Could you check a few things on this model? Use its own coordinates, in mm. Give positions to 0.01 mm unless a question says otherwise; leave off trailing zeros. Write each loop counter-clockwise with the first axis right and the second up, starting at its lowest first coordinate (ties: lowest second). Pieces come first, ordered by that corner, then holes. Notation, with made-up numbers: (-27, 47) - (12, 47) arc R32 ccw to (12, 83) - close; hole circle Ø10 at (23.25, 56.25). An arc over 180 degrees is marked (long way). Answer as a JSON object with one key per item and string values. Group by question number.
```python
from build123d import *

# Parameters (mm, degrees)
ESQUISSE1_R        = 2
ESQUISSE1_R_2      = 1.5
BOSS_EXTRU_1_DEPTH = 2.5


with BuildPart() as part:
    # Esquisse1 → Boss.-Extru.1 (new body)
    with BuildSketch(Plane.XY):
        with BuildLine():
            Line((0, 0), (70, 0))
            Line((70, 0), (70, 10))
            Line((70, 10), (0, 10))
            ThreePointArc((0, 10), (-8.007101932, 13.316650215), (-11.323752147, 21.323752147))
            Line((-11.323752147, 21.323752147), (-11.323752147, 31.323752147))
            Line((-11.323752147, 31.323752147), (-21.323752147, 31.323752147))
            Line((-21.323752147, 31.323752147), (-21.323752147, 21.323752147))
            ThreePointArc((-21.323752147, 21.323752147), (-15.078169744, 6.245582404), (0, 0))
        make_face()
        with Locations((-16.323752147, 26.323752147)):
            Circle(ESQUISSE1_R, mode=Mode.SUBTRACT)
        with Locations((66.53, 5)):
            Circle(ESQUISSE1_R_2, mode=Mode.SUBTRACT)
        with Locations((53.31, 5)):
            Circle(ESQUISSE1_R_2, mode=Mode.SUBTRACT)
    extrude(amount=BOSS_EXTRU_1_DEPTH)


solid = part.part
```
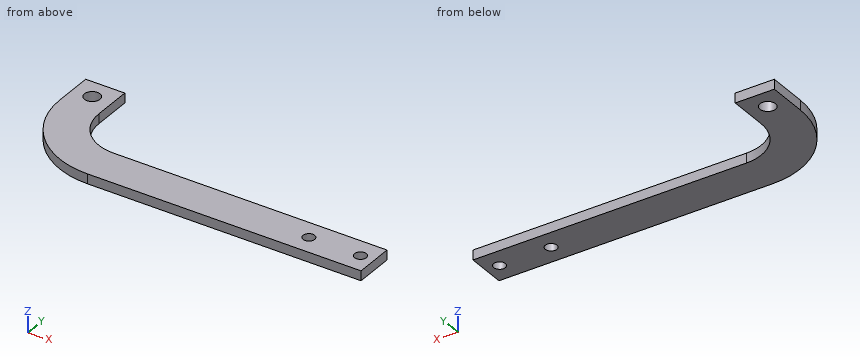
(1) I want a section at B-B, the plane z = 1.2. Please give me the cut outline in (x, y), and give its area (3 significant figures).
(2) I want a section at C-C, the plane y = 5. Please give me the cut outline in (x, z).
(3) I need wall thicknesses on L1, parallel to X at y = 6, z = 1.8; L2, parallel to Y at x = 66.53, z = 1.9; L3, parallel to X at y = 5.5, z = 2.15. Which ranges of each line are inside material? Lowest first, please.
(4) I want a section at D-D, the plane x = 50.5. Please give me the cut outline in (y, z).
(5) Will these pins go through, and if not, where does the flat tip stop? P1, Ø2.5, axis at x = 66.53, y = 5, coming from the +Z side; P2, Ø1.2, axis at y = 28.5, z = 1, coming from the +X side.
(6) I want a section at A-A, the plane x = 66.53. Please give me the cut outline in (y, z), and give its area (3 significant figures).
Entries:
{
 "1": {"outline": "(-21.32, 21.32) arc R21.32 ccw to (0, 0) - (70, 0) - (70, 10) - (0, 10) arc R11.32 cw to (-11.32, 21.32) - (-11.32, 31.32) - (-21.32, 31.32) - close; hole circle Ø4 at (-16.32, 26.32); hole circle Ø3 at (53.31, 5); hole circle Ø3 at (66.53, 5)", "area": "1,030 mm^2"},
 "2": {"outline": "(-13.72, 0) - (51.81, 0) - (51.81, 2.5) - (-13.72, 2.5) - close; (54.81, 0) - (65.03, 0) - (65.03, 2.5) - (54.81, 2.5) - close; (68.03, 0) - (70, 0) - (70, 2.5) - (68.03, 2.5) - close"},
 "3": {"L1": "-14.83 to 52.19, 54.43 to 65.41, 67.65 to 70", "L2": "0 to 3.5, 6.5 to 10", "L3": "-14.29 to 51.9, 54.72 to 65.12, 67.94 to 70"},
 "4": {"outline": "(0, 0) - (10, 0) - (10, 2.5) - (0, 2.5) - close"},
 "5": {"P1": "through", "P2": "x = -11.32"},
 "6": {"outline": "(0, 0) - (3.5, 0) - (3.5, 2.5) - (0, 2.5) - close; (6.5, 0) - (10, 0) - (10, 2.5) - (6.5, 2.5) - close", "area": "17.5 mm^2"}
}
